```python
from build123d import *

# Parameters (mm, degrees)
EXTRUDE1_DEPTH = 0.1905
FILLET1_R      = 0.762


with BuildPart() as part:
    # Sketch1 → Extrude1 (new body, symmetric)
    with BuildSketch(Plane(origin=(0, 0, 0), x_dir=(0, 0, -1), z_dir=(1, 0, 0))):
        with BuildLine():
            Line((0.059401011, 3.403081615), (1.01175594, 3.386458198))
            Line((1.01175594, 3.386458198), (1.337932753, 2.159059043))
            ThreePointArc((1.337932753, 2.159059043), (0, -2.7686), (-1.337932753, 2.159059043))
            Line((-1.337932753, 2.159059043), (-1.01175594, 3.386458198))
            Line((-1.01175594, 3.386458198), (-0.059401011, 3.403081615))
            Line((-0.059401011, 3.403081615), (-0.053859872, 3.085629972))
            Line((-0.053859872, 3.085629972), (-0.291948604, 3.081474118))
            ThreePointArc((-0.291948604, 3.081474118), (-0.603859108, 2.758481335), (-0.280866326, 2.446570831))
            Line((-0.280866326, 2.446570831), (-0.042777593, 2.450726686))
            Line((-0.042777593, 2.450726686), (-0.037236454, 2.133275042))
            ThreePointArc((-0.037236454, 2.133275042), (0, -2.1336), (0.037236454, 2.133275042))
            Line((0.037236454, 2.133275042), (0.042777593, 2.450726686))
            Line((0.042777593, 2.450726686), (0.280866326, 2.446570831))
            ThreePointArc((0.280866326, 2.446570831), (0.603859108, 2.758481335), (0.291948604, 3.081474118))
            Line((0.291948604, 3.081474118), (0.053859872, 3.085629972))
            Line((0.053859872, 3.085629972), (0.059401011, 3.403081615))
        make_face()
    extrude(amount=EXTRUDE1_DEPTH, both=True)

    # Fillet1
    fillet1_edges = [part.edges().sort_by_distance(p)[0] for p in [
        (0, 3.386458198, -1.01175594),
        (0, 2.159059043, -1.337932753),
        (0, 2.159059043, 1.337932753),
        (0, 3.386458198, 1.01175594),
    ]]
    fillet(fillet1_edges, radius=FILLET1_R)


solid = part.part
```
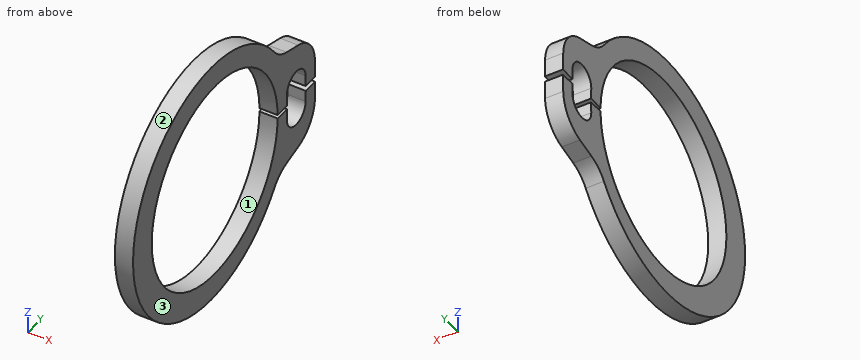
CAD build for the part. Positions are in the model's coordinates, mm. Face numbers are marked on the shaded views. Round coordinates to 2 decimals unless told otherwise and drop trailing zeros. Order: outer loops, then holes, each group sorted by start corner. A loop starts at its lowest first (then second) coordinate and runs counter-clockwise, first axis right, second up. Notation, with made-up numbers: (87.25, -13) -> (112.25, -13) arc R6 cw to (112.25, -7) -> close; hole circle Ø3 at (63.25, -8). An arc over 180 degrees is marked (long way). One line per question, with ' | ' between items.
Q1. Two-plate mould, pull along Z, no slides. Class the marked faces 1, 2 and 3: released by +Z, released by -Z, zero draft, split by the parting line, or undercut.
Completed:
face 1: undercut | face 2: split by the parting line | face 3: zero draft
Q2. Probe probe 1 along Y at (x, z) = (-0.05, 0.75); probe 2 along Y at (x, z) = (0.1, 1.5); probe 3 along Z at (x, y) = (-0.05, 0). List the from-to ranges inside material, lowest first.
Completed:
probe 1: y = -2.66 to -2, 2 to 3.32 | probe 2: y = -2.3 to -1.52, 1.52 to 2.06 | probe 3: z = -2.64 to -2.13, 2.13 to 2.64
Q3. Slice it at B-B (z = 1.9). Write the cut outline in (x, y), then the cut area to 3 significant figures.
Completed:
outline: (-0.19, -1.96) -> (0.19, -1.96) -> (0.19, -0.97) -> (-0.19, -0.97) -> close; (-0.19, 0.97) -> (0.19, 0.97) -> (0.19, 1.72) -> (-0.19, 1.72) -> close | area: 0.663 mm^2
Q4. Slice it at A-A (y = 2.75). Write the cut outline in (x, z), then the cut area to 3 significant figures.
Completed:
outline: (-0.19, -1.18) -> (0.19, -1.18) -> (0.19, -0.6) -> (-0.19, -0.6) -> close; (-0.19, 0.6) -> (0.19, 0.6) -> (0.19, 1.18) -> (-0.19, 1.18) -> close | area: 0.440 mm^2
